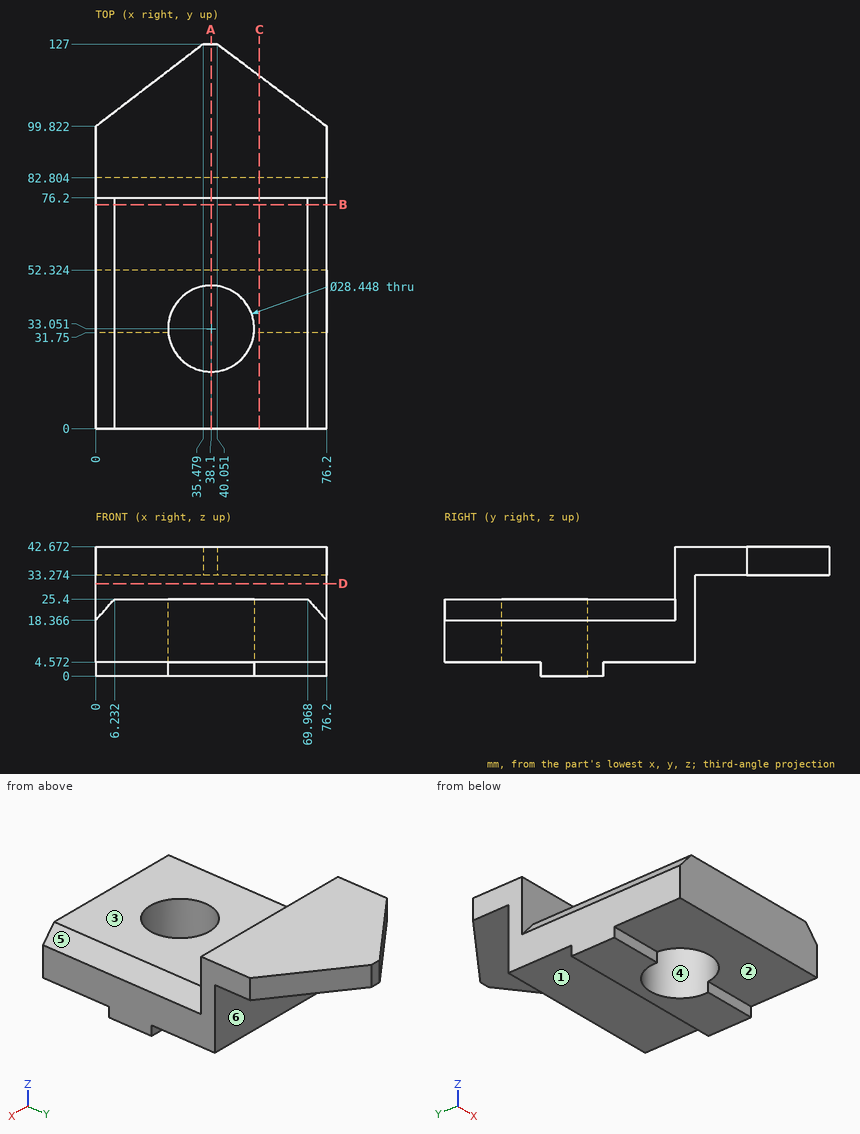
The drawing under review shows one solid part. Ordinate dimensions are in mm from its lowest x, y, z. A direction names the side the tool comes from. Round coordinates to 2 decimals unless told otherwise and drop trailing zeros. Write each loop counter-clockwise with the first axis right and the second up, starting at its lowest first coordinate (ties: lowest second). Pieces come first, ordered by that corner, then holes. Notation, with made-up numbers: (79.25, -26.5) -> (128.25, -26.5) arc R33 cw to (128.25, 12.5) -> close; hole circle Ø4 at (13, -30). An arc over 180 degrees is marked (long way). One line per question, with ' | ' between items.
(1) Take a section at C-C, the plane x = 54. State the section outline as (y, z) points.
Result sheet:
outline: (0, 4.57) -> (31.75, 4.57) -> (31.75, 0) -> (52.32, 0) -> (52.32, 4.57) -> (82.8, 4.57) -> (82.8, 33.27) -> (116.51, 33.27) -> (116.51, 42.67) -> (76.2, 42.67) -> (76.2, 25.4) -> (0, 25.4) -> close
(2) Wall thickness on line 1 (Y direction, x = 38.1, z = 20.25) (1 decimal); line 2 (Z direction, x = 65, y = 72.5); line 3 (Z direction, x = 41, y = 79.5): over which ranges is each line inside the solid? List them lowest first. Write a range as [from, to].
Result sheet:
line 1: [0, 18.8], [47.3, 82.8] | line 2: [4.57, 25.4] | line 3: [4.57, 42.67]
(3) Machinability: for the marked faces 1, 2 and 3, which of the approach directions +Z, -Z, +X, -X, +Y, -Y give a long, thin tool a straight path to every point of the face, cutting with its end or side? Answer none if there is none.
Result sheet:
face 1: -Z, +X, -X, +Y | face 2: -Z, +X, -X, -Y | face 3: +Z, +X, -X, -Y
(4) Draft analysis for pull direction X (two halves, no side actions). For the marked faces 4, 5 and 6, state which applies: released by +X, released by -X, zero draft, split by the parting line, or undercut.
Result sheet:
face 4: undercut | face 5: released by +X | face 6: zero draft
(5) Insertion check: P1, Ø1, axis at x = 38.5, z = 4.5, coming from the +Y side; P2, Ø8, axis at x = 10, y = 25.5, coming from the -Z side; P3, Ø5, axis at x = 64, z = 2, coming from the -Y side. Each pin has a flat end and moves straight along its axis. Give the tip position at first contact, or say it passes through.
Result sheet:
P1: y = 82.8 | P2: z = 4.57 | P3: y = 31.75
(6) Take a section at A-A, the plane x = 38.1. State the section outline as (y, z) points (1 decimal).
Result sheet:
outline: (0, 4.6) -> (18.8, 4.6) -> (18.8, 25.4) -> (0, 25.4) -> close; (47.3, 0) -> (52.3, 0) -> (52.3, 4.6) -> (82.8, 4.6) -> (82.8, 33.3) -> (127, 33.3) -> (127, 42.7) -> (76.2, 42.7) -> (76.2, 25.4) -> (47.3, 25.4) -> close
(7) Take a section at B-B, the plane y = 74. State the section outline as (x, z) points (1 decimal).
Result sheet:
outline: (0, 4.6) -> (76.2, 4.6) -> (76.2, 18.4) -> (70, 25.4) -> (6.2, 25.4) -> (0, 18.4) -> close
(8) Take a section at D-D, the plane z = 30.5. State the section outline as (x, y) points.
Result sheet:
outline: (0, 76.2) -> (76.2, 76.2) -> (76.2, 82.8) -> (0, 82.8) -> close
